Design review of the part built by this model. Coordinates are the model's own, in mm. Face numbers are marked on the shaded views. A direction names the side the tool comes from. Round coordinates to 2 decimals unless told otherwise and drop trailing zeros. Loops run counter-clockwise (first coordinate to the right, second up) from the corner with the lowest first, then second, coordinate; pieces in that order, holes last. Notation, with made-up numbers: (36, 4.25) - (45, 4.25) arc R17 cw to (45, 24.25) - close; hole circle Ø2 at (49.25, -5.5). An arc over 180 degrees is marked (long way). Return JSON: item names as keys, results as strings. Group by question number.
(1) For the marked faces 4 and 5, list the 3-axis set-ups (+Z, -Z, +X, -X, +Y, -Y) from which the entire face can be reached by the end or side of a thin tool; tool diameter is ignored.
(2) We need section A-A, the plane x = -75.5. Write out the cut boundary in (y, z).
(3) Wall thickness on L1, parallel to Z at x = -75.5, y = -8; L2, parallel to Y at x = 40, z = 8.75; L3, parallel to X at y = 0, z = 13.25: over which ranges is each line inside the solid? List them lowest first. Write a range as [from, to].
(4) We need section B-B, the plane z = 9.5. Give the number of separate pieces and of enclosed holes in the cut face, and give its area (3 significant figures).
(5) Clearance check with flat-ended pins moving along their axes: pin 1 (7 mm diameter, centred on x = -75.5, z = 9.5, fed in from +Y); pin 2 (4 mm diameter, centred on y = 22.5, z = 8, fed in from +X); pin 3 (7.5 mm diameter, centred on x = 73, z = 12, fed in from +Y); pin 4 (3.5 mm diameter, centred on x = 77, z = 9.5, fed in from +Y). State where each tip first meets the part, or that it passes through.
(6) The part is to be moulded in two halves that separate along Y. For the marked faces 1, 2 and 3, say which applies: pulls with the +Y half, pulls with the -Y half, needs draft (parallel to the pull), parting line crosses it, or undercut.
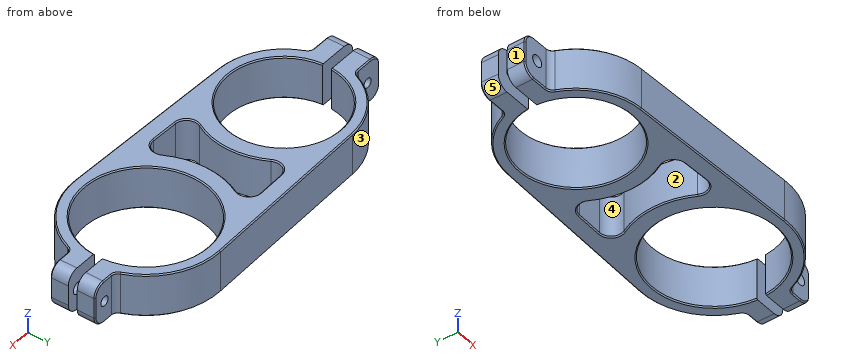
from build123d import *

# Parameters (mm, degrees)
F1_DEPTH = 19
F2_R     = 2.1
F3_DEPTH = 25
F4_R     = 2.6
F5_DEPTH = 10
F6_R     = 2.6
F7_DEPTH = 10
F8_R     = 5
F9_SIZE  = 0.5
F10_SIZE = 0.5
F11_R    = 3
F12_SIZE = 0.5


with BuildPart() as f1:
    # F0 (on Top) → F1 (new body)
    with BuildSketch(Plane.XY):
        with BuildLine():
            ThreePointArc((-64.919872, 2), (-15, 0), (-64.919872, -2))
            Line((-64.919872, -2), (-82.5, -2))
            Line((-82.5, -2), (-82.5, -10))
            Line((-82.5, -10), (-68.284271, -10))
            ThreePointArc((-68.284271, -10), (-57.701173, -24.22124), (-40.9375, -29.985348))
            Line((-40.9375, -29.985348), (38.984375, -32.484127))
            ThreePointArc((38.984375, -32.484127), (58.708317, -26.575343), (70.923292, -10))
            Line((70.923292, -10), (82.5, -10))
            Line((82.5, -10), (82.5, -2))
            Line((82.5, -2), (67.427176, -2))
            ThreePointArc((67.427176, -2), (12.5, 0), (67.427176, 2))
            Line((67.427176, 2), (82.5, 2))
            Line((82.5, 2), (82.5, 10))
            Line((82.5, 10), (70.923292, 10))
            ThreePointArc((70.923292, 10), (58.708317, 26.575343), (38.984375, 32.484127))
            Line((38.984375, 32.484127), (-40.9375, 29.985348))
            ThreePointArc((-40.9375, 29.985348), (-57.701173, 24.22124), (-68.284271, 10))
            Line((-68.284271, 10), (-82.5, 10))
            Line((-82.5, 10), (-82.5, 2))
            Line((-82.5, 2), (-64.919872, 2))
        make_face()
        with BuildLine():
            ThreePointArc((-7.553076, -23.525456), (-11.757166, -20.974822), (-11.743915, -16.057512))
            ThreePointArc((-11.743915, -16.057512), (-7.5, 0), (-11.743915, 16.057512))
            ThreePointArc((-11.743915, 16.057512), (-11.757166, 20.974822), (-7.553076, 23.525456))
            Line((-7.553076, 23.525456), (4.594653, 23.905258))
            ThreePointArc((4.594653, 23.905258), (9.00079, 21.541796), (9.15704, 16.544238))
            ThreePointArc((9.15704, 16.544238), (5, 0), (9.15704, -16.544238))
            ThreePointArc((9.15704, -16.544238), (9.00079, -21.541796), (4.594653, -23.905258))
            Line((4.594653, -23.905258), (-7.553076, -23.525456))
        make_face(mode=Mode.SUBTRACT)
    extrude(amount=F1_DEPTH)

    # F2 (on face) → F3 (cut)
    with BuildSketch(Plane.XZ.offset(10)):
        with Locations((-75.5, 9.5)):
            Circle(F2_R)
        with Locations((77, 9.5)):
            Circle(F2_R)
    extrude(amount=-F3_DEPTH, mode=Mode.SUBTRACT)

    # F4 (on face) → F5 (cut)
    with BuildSketch(Plane.XZ.offset(10)):
        with Locations((-75.5, 9.5)):
            Circle(F4_R)
    extrude(amount=-F5_DEPTH, mode=Mode.SUBTRACT)

    # F6 (on face) → F7 (cut)
    with BuildSketch(Plane.XZ.offset(10)):
        with Locations((77, 9.5)):
            Circle(F6_R)
    extrude(amount=-F7_DEPTH, mode=Mode.SUBTRACT)

    # F8
    f8_edges = [f1.edges().sort_by_distance(p)[0] for p in [
        (82.5, 6, 19),
        (82.5, -6, 19),
        (82.5, 6, 0),
        (82.5, -6, 0),
        (-82.5, -6, 0),
        (-82.5, -6, 19),
        (-82.5, 6, 19),
        (-82.5, 6, 0),
    ]]
    fillet(f8_edges, radius=F8_R)

    # F9
    f9_edges = [f1.edges().sort_by_distance(p)[0] for p in [
        (-15, 0, 0),
        (12.5, 0, 0),
        (12.5, 0, 19),
        (-15, 0, 19),
    ]]
    chamfer(f9_edges, length=F9_SIZE)

    # F10
    f10_edges = [f1.edges().sort_by_distance(p)[0] for p in [
        (-1.479211, 23.715357, 19),
        (5, 0, 0),
    ]]
    chamfer(f10_edges, length=F10_SIZE)

    # F11
    f11_edges = [f1.edges().sort_by_distance(p)[0] for p in [
        (-68.284271, 10, 9.5),
        (-68.284271, -10, 9.5),
        (70.923292, -10, 9.5),
        (70.923292, 10, 9.5),
    ]]
    fillet(f11_edges, radius=F11_R)

    # F12
    f12_edges = [f1.edges().sort_by_distance(p)[0] for p in [
        (57.873558, 27.143801, 19),
        (57.873558, -27.143801, 19),
    ]]
    chamfer(f12_edges, length=F12_SIZE)


solid = f1.part
Solutions:
{
 "1": {"face 4": "+Z, -Z", "face 5": "-Z, -X, +Y, -Y"},
 "2": {"outline": "(-10, 0.5) - (-9.5, 0) - (-2, 0) - (-2, 6.9) - (-10, 6.9) - close; (-10, 12.1) - (-2, 12.1) - (-2, 19) - (-9.5, 19) - (-10, 18.5) - close; (2, 0) - (9.5, 0) - (10, 0.5) - (10, 7.4) - (2, 7.4) - close; (2, 11.6) - (10, 11.6) - (10, 18.5) - (9.5, 19) - (2, 19) - close"},
 "3": {"L1": "[0, 6.9], [12.1, 19]", "L2": "[-32.5, -27.5], [27.5, 32.5]", "L3": "[-15, -7.5], [5, 12.5]"},
 "4": {"separate pieces": "5", "enclosed holes": "1", "area": "3,130 mm^2"},
 "5": {"pin 1": "y = 10", "pin 2": "x = 65.22", "pin 3": "y = 14.17", "pin 4": "through"},
 "6": {"face 1": "needs draft", "face 2": "undercut", "face 3": "pulls with the +Y half"}
}
